Could you check a few things on this model? Use its own coordinates, in mm. A direction names the side the tool comes from. Round coordinates to 2 decimals unless told otherwise and drop trailing zeros. Write each loop counter-clockwise with the first axis right and the second up, starting at its lowest first coordinate (ties: lowest second). Pieces come first, ordered by that corner, then holes. Notation, with made-up numbers: (-32, -18) -> (-3, -18) arc R21 ccw to (-3, 3) -> close; hole circle Ø2 at (17, 28.25). An arc over 180 degrees is marked (long way). Answer in a Markdown table with one row per item.
from build123d import *

# Parameters (mm, degrees)
F0_W     = 57.15
F0_H     = 44.45
F1_DEPTH = 12.7
F3_DEPTH = 12.7
F5_DEPTH = 25.4


with BuildPart() as f1:
    # F0 (on Front) → F1 (new body)
    with BuildSketch(Plane.XZ):
        with Locations((28.575, 22.225)):
            Rectangle(F0_W, F0_H)
    extrude(amount=F1_DEPTH)

    # F2 (on face) → F3 (join)
    with BuildSketch(Plane.XZ.offset(12.7)):
        Polygon((19.05, 44.45), (0, 44.45), (0, 0), (44.45, 0), align=None)
    extrude(amount=F3_DEPTH)

    # F4 (on face) → F5 (cut)
    with BuildSketch(Plane.XZ.offset(25.4)):
        with BuildLine():
            ThreePointArc((34.731897, 17.00668), (37.082178, 20.914199), (37.900781, 25.4))
            ThreePointArc((37.900781, 25.4), (33.291142, 35.18959), (22.808487, 37.872647))
            Line((22.808487, 37.872647), (34.731897, 17.00668))
        make_face()
        with BuildLine():
            Line((34.731897, 17.00668), (22.808487, 37.872647))
            ThreePointArc((22.808487, 37.872647), (14.174093, 19.099035), (34.731897, 17.00668))
        make_face()
    extrude(amount=-F5_DEPTH, mode=Mode.SUBTRACT)


solid = f1.part
1) Imagine slicing it at B-B, the plane z = 24.5. Please give me the cut outline in (x, y), plus the area to 3 significant figures.
Findings:
| item | result |
|---|---|
| outline | (0, -25.4) -> (12.53, -25.4) -> (12.53, 0) -> (0, 0) -> close; (37.87, -12.7) -> (57.15, -12.7) -> (57.15, 0) -> (37.87, 0) -> close |
| area | 563 mm^2 |
2) Imagine slicing it at C-C, the plane x = 31.5. Please give me the cut outline in (y, z), plus the area to 3 significant figures.
Findings:
| item | result |
|---|---|
| outline | (-25.4, 0) -> (0, 0) -> (0, 14.37) -> (-25.4, 14.37) -> close; (-12.7, 36.43) -> (0, 36.43) -> (0, 44.45) -> (-12.7, 44.45) -> close |
| area | 467 mm^2 |
3) Imagine slicing it at D-D, the plane y = -15. Please give me the cut outline in (x, z), plus the area to 3 significant figures.
Findings:
| item | result |
|---|---|
| outline | (0, 0) -> (44.45, 0) -> (34.73, 17.01) arc R12.7 cw (long way) to (22.81, 37.87) -> (19.05, 44.45) -> (0, 44.45) -> close |
| area | 1,060 mm^2 |
4) Please list where these lines run through material, in increasing order: line 1 (X direction, y = -6.25, z = 25.4); line 2 (Z direction, x = 25, y = -11.5); line 3 (Y direction, x = 46, z = 11).
Findings:
| item | result |
|---|---|
| line 1 | x = 0 to 12.5, 37.9 to 57.15 |
| line 2 | z = 0 to 12.7, 38.1 to 44.45 |
| line 3 | y = -12.7 to 0 |
5) For pin 1 (19 mm diameter, centred on x = 33.5, z = 28.5, fed in from -Y), with a flat end and sliding along its axis, tell me the tip position at first contact or that it passes through.
Findings:
| item | result |
|---|---|
| pin 1 | stops at y = -12.7 |
6) For faces 1 (the face through (23, -10, 44.45)), 2 (the face through (39.66, -18.96, 8.38)), which set-ups out of +Z, -Z, +X, -X, +Y, -Y let a thin tool reach every point of the face, with its end or its side?
Findings:
| item | result |
|---|---|
| face 1 | +Z, +X, -X, +Y, -Y |
| face 2 | +Z, +X, -Y |
7) Imagine slicing it at A-A, the plane y = -9.5. Please give me the cut outline in (x, z), plus the area to 3 significant figures.
Findings:
| item | result |
|---|---|
| outline | (0, 0) -> (57.15, 0) -> (57.15, 44.45) -> (0, 44.45) -> close; hole (22.81, 37.87) arc R12.7 ccw (long way) to (34.73, 17.01) arc R12.7 ccw to (37.9, 25.4) arc R12.7 ccw to start |
| area | 2,030 mm^2 |
